Can you work these out from the model? Positions are in its coordinate system, mm. Face numbers are marked on the shaded views. A direction names the side the tool comes from. Coordinates: 2 decimals unless noted, no trailing zeros. Order: outer loops, then holes, each group sorted by start corner. A loop starts at its lowest first (then second) coordinate and runs counter-clockwise, first axis right, second up. Notation, with made-up numbers: (-16.5, 80) - (-8.5, 80) arc R21 ccw to (-8.5, 92) - close; hole circle Ø8 at (-15.5, 36.25). An arc over 180 degrees is marked (long way). Use a Markdown table: item, result. Add a question column.
(1) For pin 1 Ø2 at (x, z) = (-2, 9.5) entering from +Y, with a flat end and sliding along its axis, tell me the tip position at first contact or that it passes through.
(2) I want a section at A-A (z = -1.25). List the corners of the cut face in (x, y) for me, and give its area (3 significant figures).
(3) We'd pull the mould along X, two halves only. Please class the marked faces 1 and 2: pulls with the +X half, pulls with the -X half, needs draft (parallel to the pull), parting line crosses it, or undercut.
(4) If I drill on L1, parallel to Y at x = -0.15, z = 4.5; L2, parallel to Z at x = 1.95, y = 1.5, over which ranges is the centre line in solid material (lowest first)? Write a range as [from, to].
(5) On a 3-axis mill with a long thin cutter (end or side, diameter ignored), from which of +Z, -Z, +X, -X, +Y, -Y can I reach the whole of each face in a straight line? I mean the marked faces 3 and 4. Say none if no direction works.
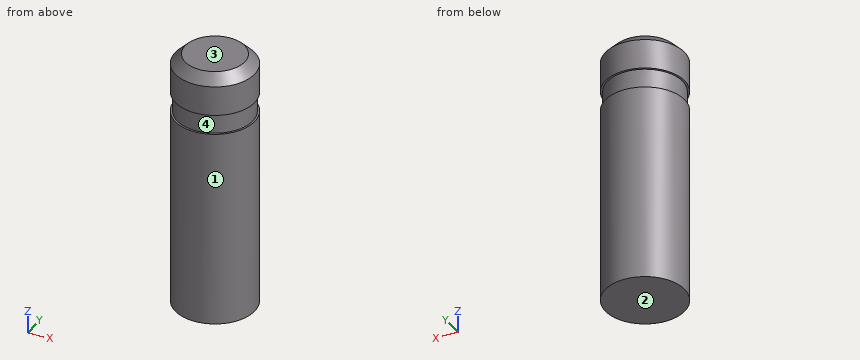
```python
from build123d import *

# Parameters (mm, degrees)
SKETCH1_R           = 2
BOSS_EXTRUDE1_DEPTH = 13
CUT_EXTRUDE1_START  = -10
SKETCH2_OUTSIDE_W   = 8.836
SKETCH2_OUTSIDE_H   = 8.836
SKETCH2_OUTSIDE_R   = 1.9
CUT_EXTRUDE1_DEPTH  = 1
CHAMFER1_SIZE       = 0.5
SCALE1_SCALE        = 1.5


with BuildPart() as part:
    # Sketch1 → Boss-Extrude1 (new body)
    with BuildSketch(Plane.XY):
        with Locations(Location((0, 0, 0), (0, 0, 180))):
            Circle(SKETCH1_R)
    extrude(amount=BOSS_EXTRUDE1_DEPTH)

    # Sketch2 outside → Cut-Extrude1 (cut)
    with BuildSketch(Plane(origin=(0, 0, 0), x_dir=(-1, 0, 0), z_dir=(0, 0, -1)).offset(CUT_EXTRUDE1_START)):
        Rectangle(SKETCH2_OUTSIDE_W, SKETCH2_OUTSIDE_H)
        Circle(SKETCH2_OUTSIDE_R, mode=Mode.SUBTRACT)
    extrude(amount=-CUT_EXTRUDE1_DEPTH, mode=Mode.SUBTRACT)

    # Chamfer1
    chamfer1_edges = [part.edges().sort_by_distance(p)[0] for p in [
        (2, 0, 13),
    ]]
    chamfer(chamfer1_edges, length=CHAMFER1_SIZE)


with BuildPart() as part_1:
    # Scale1: scaled about (0, 0, 6.412787951)
    add(part.part.scale(SCALE1_SCALE).moved(Location((0, 0, -3.206393976))))


solid = part_1.part
```
Answers follow:
| question | item | result |
|---|---|---|
| 1 | pin 1 | stops at y = 2.83 |
| 2 | outline | circle Ø6 at (0, 0) |
| 2 | area | 28.3 mm² |
| 3 | face 1 | parting line crosses it |
| 3 | face 2 | needs draft |
| 4 | L1 | y = [-3, 3] |
| 4 | L2 | z = [-3.21, 16.08] |
| 5 | face 3 | +Z, +X, -X, +Y, -Y |
| 5 | face 4 | none |
